Input: part model. Units: mm. Frame: model coordinates. Round coordinates to 2 decimals unless told otherwise and drop trailing zeros. Loops run counter-clockwise (first coordinate to the right, second up) from the corner with the lowest first, then second, coordinate; pieces in that order, holes last.
1) Draft query along Z for faces 1 (the face through (-7.559, -12.522, -5.796)), 2 (the face through (0, -13, -25.4)), 3 (the face through (12.88, -12.52, 39.4)). Return one class per face: pulls with the +Z half, pulls with the -Z half, needs draft (parallel to the pull), parting line crosses it, or undercut.
2) Section C-C, the plane y = -5. Return loops of the section in (x, z) (3 decimals), and give its area (3 significant figures).
3) Section A-A, the plane z = 0. Return loops of the section in (x, y) (3 decimals).
4) Section D-D, the plane x = 14. Return loops of the section in (y, z), and give its area (3 significant figures).
5) First-contact query: pin 1 (17 mm diameter, centred on x = 0, z = 0, fed in from -Y); pin 2 (1 mm diameter, centred on x = -18.5, y = -15.5, fed in from +Z). Flat tips, straight axial feed; report the tip coordinate or a pass-through.
6) Section B-B, the plane x = 3.5. Return loops of the section in (y, z), and give its area (3 significant figures).
7) Ray query, line 1 along Z through (x, y) = (0, -19) (3 decimals); line 2 along X through (y, z) = (-11.5, -4.5); line 3 along Z through (x, y) = (2, -16.5). Return the intervals inside material, ascending.
from build123d import *

# Parameters (mm, degrees)
F0_W     = 50.8
F0_H     = 50.8
F0_R     = 9.525
F1_DEPTH = 25.4


with BuildPart() as f1:
    # F0 (on Front) → F1 (new body)
    with BuildSketch(Plane.XZ):
        Rectangle(F0_W, F0_H)
        Circle(F0_R, mode=Mode.SUBTRACT)
        Polygon((0, 53.798063), (-25.4, 25.4), (25.4, 25.4), align=None)
    extrude(amount=F1_DEPTH)


solid = f1.part
Final values:
1. face 1: undercut
1. face 2: pulls with the -Z half
1. face 3: pulls with the +Z half
2. outline: (-25.4, -25.4) - (25.4, -25.4) - (25.4, 25.4) - (0, 53.798) - (-25.4, 25.4) - close; hole circle Ø19.05 at (0, 0)
2. area: 3,020 mm2
3. outline: (-25.4, -25.4) - (-9.525, -25.4) - (-9.525, 0) - (-25.4, 0) - close; (9.525, -25.4) - (25.4, -25.4) - (25.4, 0) - (9.525, 0) - close
4. outline: (-25.4, -25.4) - (0, -25.4) - (0, 38.15) - (-25.4, 38.15) - close
4. area: 1,610 mm2
5. pin 1: passes through
5. pin 2: stops at z = 33.67
6. outline: (-25.4, -25.4) - (0, -25.4) - (0, -8.86) - (-25.4, -8.86) - close; (-25.4, 8.86) - (0, 8.86) - (0, 49.88) - (-25.4, 49.88) - close
6. area: 1,460 mm2
7. line 1: z = -25.4 to -9.525, 9.525 to 53.798
7. line 2: x = -25.4 to -8.39, 8.39 to 25.4
7. line 3: z = -25.4 to -9.31, 9.31 to 51.56
